For this review, take the finished solid that the model builds, in its own axes (mm). Coordinates: 2 decimals unless noted, no trailing zeros. Loops run counter-clockwise (first coordinate to the right, second up) from the corner with the lowest first, then second, coordinate; pieces in that order, holes last. Notation, with made-up numbers: M -7,-5 L 44,-5 A23 ccw 44,17 Z; hole C 76.5,52.5 d3. An arc over 180 degrees is marked long. Write item = value, one per line.
from build123d import *

# Parameters (mm, degrees)
SKETCH1_W           = 127
SKETCH1_H           = 127
BOSS_EXTRUDE1_DEPTH = 3.175
SKETCH2_R           = 11.1125
SKETCH2_R_2         = 8.73125
CUT_EXTRUDE1_DEPTH  = 3.175
SKETCH3_R           = 4.7625
CUT_EXTRUDE2_DEPTH  = 3.175


with BuildPart() as part:
    # Sketch1 → Boss-Extrude1 (new body)
    with BuildSketch(Plane.XY):
        Rectangle(SKETCH1_W, SKETCH1_H)
    extrude(amount=BOSS_EXTRUDE1_DEPTH)

    # Sketch2 → Cut-Extrude1 (cut)
    with BuildSketch(Plane(origin=(0, 0, 0), x_dir=(-1, 0, 0), z_dir=(0, 0, -1))):
        with Locations((0, 25.4)):
            Circle(SKETCH2_R)
        with Locations((31.75, 25.4)):
            Circle(SKETCH2_R_2)
        with Locations((0, -25.4)):
            Circle(SKETCH2_R)
    extrude(amount=-CUT_EXTRUDE1_DEPTH, mode=Mode.SUBTRACT)

    # Sketch3 → Cut-Extrude2 (cut)
    with BuildSketch(Plane(origin=(0, 0, 0), x_dir=(-1, 0, 0), z_dir=(0, 0, -1))):
        with Locations((52.3875, 52.3875)):
            Circle(SKETCH3_R)
        with Locations(Location((52.3875, -52.3875, 0), (0, 0, 180))):
            Circle(SKETCH3_R)
        with Locations(Location((-52.3875, 52.3875, 0), (0, 0, 180))):
            Circle(SKETCH3_R)
        with Locations((-52.3875, -52.3875)):
            Circle(SKETCH3_R)
    extrude(amount=-CUT_EXTRUDE2_DEPTH, mode=Mode.SUBTRACT)


solid = part.part
Q1. Add section B-B (y = 25.4). Write out the cut boundary in (x, z) (1 decimal).
Solved:
outline = M -63.5,0 L -40.5,0 L -40.5,3.2 L -63.5,3.2 Z; M -23,0 L -11.1,0 L -11.1,3.2 L -23,3.2 Z; M 11.1,0 L 63.5,0 L 63.5,3.2 L 11.1,3.2 Z
Q2. Add section A-A (x = 0). Write out the cut boundary in (y, z) (1 decimal).
Solved:
outline = M -63.5,0 L -36.5,0 L -36.5,3.2 L -63.5,3.2 Z; M -14.3,0 L 14.3,0 L 14.3,3.2 L -14.3,3.2 Z; M 36.5,0 L 63.5,0 L 63.5,3.2 L 36.5,3.2 Z
Q3. Add section D-D (y = -25.4). Write out the cut boundary in (x, z) (1 decimal), and give its area (3 significant figures).
Solved:
outline = M -63.5,0 L -11.1,0 L -11.1,3.2 L -63.5,3.2 Z; M 11.1,0 L 63.5,0 L 63.5,3.2 L 11.1,3.2 Z
area = 333 mm²
Q4. For line 1 along Y through (x, z) = (0, 1.4); line 2 along Y through (x, z) = (-53, 0.75); line 3 along X through (y, z) = (29, 1.9), list the stretches that pass through material, from the lowest coordinate up.
Solved:
line_1 = -63.5 to -36.51, -14.29 to 14.29, 36.51 to 63.5
line_2 = -63.5 to -57.11, -47.66 to 47.66, 57.11 to 63.5
line_3 = -63.5 to -39.7, -23.8 to -10.51, 10.51 to 63.5
Q5. Draft analysis for pull direction X (two halves, no side actions). For faces 1 (the face through (-1, 1, 3.175)), 2 (the face through (63.5, -1, 2)), 3 (the face through (47.63, 52.18, 1.57)), state which applies: +X half, -X half, draft (parallel to the pull), parting line (faces both ways), or undercut.
Solved:
face_1 = draft
face_2 = +X half
face_3 = undercut
Q6. Add section C-C (x = -31.75). Write out the cut boundary in (y, z) (3 decimals), and give its area (3 significant figures).
Solved:
outline = M -63.5,0 L 16.669,0 L 16.669,3.175 L -63.5,3.175 Z; M 34.131,0 L 63.5,0 L 63.5,3.175 L 34.131,3.175 Z
area = 348 mm²
